from build123d import *

# Parameters (mm, degrees)
SKETCH1_W           = 200
SKETCH1_H           = 100
BOSS_EXTRUDE1_DEPTH = 20
SKETCH2_R           = 7.5
CUT_EXTRUDE1_DEPTH  = 20
BOSS_EXTRUDE2_DEPTH = 10
SKETCH4_R           = 7.5
CUT_EXTRUDE2_DEPTH  = 20


with BuildPart() as part:
    # Sketch1 → Boss-Extrude1 (new body)
    with BuildSketch(Plane(origin=(0, 0, 0), x_dir=(1, 0, 0), z_dir=(0, 1, 0))):
        Rectangle(SKETCH1_W, SKETCH1_H)
    extrude(amount=BOSS_EXTRUDE1_DEPTH)

    # Sketch2 → Cut-Extrude1 (cut)
    with BuildSketch(Plane(origin=(0, 20, 0), x_dir=(1, 0, 0), z_dir=(0, 1, 0))):
        with Locations((-75, 30)):
            Circle(SKETCH2_R)
        with Locations((-25, 30)):
            Circle(SKETCH2_R)
        with Locations((25, 30)):
            Circle(SKETCH2_R)
        with Locations((75, 30)):
            Circle(SKETCH2_R)
        with Locations((-75, -30)):
            Circle(SKETCH2_R)
        with Locations((-25, -30)):
            Circle(SKETCH2_R)
        with Locations((25, -30)):
            Circle(SKETCH2_R)
        with Locations((75, -30)):
            Circle(SKETCH2_R)
    extrude(amount=-CUT_EXTRUDE1_DEPTH, mode=Mode.SUBTRACT)

    # Sketch3 → Boss-Extrude2 (add, symmetric)
    with BuildSketch(Plane.XY):
        with BuildLine():
            Line((-100, 20), (100, 20))
            Line((100, 20), (157.3406431, 60.150350545))
            ThreePointArc((157.3406431, 60.150350545), (161.735357089, 79.923793338), (142.426691144, 86.045718717))
            Line((142.426691144, 86.045718717), (15.876102092, 27.36202298))
            ThreePointArc((15.876102092, 27.36202298), (0, 37.5), (-15.876102092, 27.36202298))
            Line((-15.876102092, 27.36202298), (-142.426691144, 86.045718717))
            ThreePointArc((-142.426691144, 86.045718717), (-161.735357089, 79.923793338), (-157.3406431, 60.150350545))
            Line((-157.3406431, 60.150350545), (-100, 20))
        make_face()
    extrude(amount=BOSS_EXTRUDE2_DEPTH, both=True)

    # Sketch4 → Cut-Extrude2 (cut)
    with BuildSketch(Plane.XY.offset(10)):
        with Locations((148.736996555, 72.437631209)):
            Circle(SKETCH4_R)
        with Locations((-148.736996555, 72.437631209)):
            Circle(SKETCH4_R)
    extrude(amount=-CUT_EXTRUDE2_DEPTH, mode=Mode.SUBTRACT)


solid = part.part
Can you work these out from the model? Positions are in its coordinate system, mm. A direction names the side the tool comes from. Coordinates: 2 decimals unless noted, no trailing zeros. Write each loop counter-clockwise with the first axis right and the second up, starting at its lowest first coordinate (ties: lowest second). Pieces come first, ordered by that corner, then holes. Notation, with made-up numbers: M -34.5,-2 L -0.5,-2 A31 cw -0.5,22 Z; hole C 11,-37.5 d2. An arc over 180 degrees is marked long. Use one line per item in the form item = value.
Q1. If we section it at D-D (x = -75): Write out the boundary of the cut face in (y, z), then the cut area to 3 significant figures.
Model answer:
outline = M 0,-50 L 20,-50 L 20,-37.5 L 0,-37.5 Z; M 0,-22.5 L 20,-22.5 L 20,-10 L 54.78,-10 L 54.78,10 L 20,10 L 20,22.5 L 0,22.5 Z; M 0,37.5 L 20,37.5 L 20,50 L 0,50 Z
area = 2,100 mm^2
Q2. We'd pull the mould along X, two halves only. Please class faces 6 (the cylindrical face through (-30.952, 10.14, 34.564)), 7 (the flat face through (-1, 10, 50)), 8 (the flat face through (128.269, 39.794, 0.14)), 9 (the cylindrical face through (-80.952, 10.14, -25.436)): +X half, -X half, draft (parallel to the pull), parting line (faces both ways), or undercut.
Model answer:
face_6 = undercut
face_7 = draft
face_8 = +X half
face_9 = undercut
Q3. If we section it at A-A (z = 30): Write out the boundary of the cut face in (x, y), then the cut area to 3 significant figures.
Model answer:
outline = M -100,0 L -82.5,0 L -82.5,20 L -100,20 Z; M -67.5,0 L -32.5,0 L -32.5,20 L -67.5,20 Z; M -17.5,0 L 17.5,0 L 17.5,20 L -17.5,20 Z; M 32.5,0 L 67.5,0 L 67.5,20 L 32.5,20 Z; M 82.5,0 L 100,0 L 100,20 L 82.5,20 Z
area = 2,800 mm^2
Q4. If we section it at C-C (x = 41): Write out the boundary of the cut face in (y, z), then the cut area to 3 significant figures.
Model answer:
outline = M 0,-50 L 20,-50 L 20,-10 L 39.01,-10 L 39.01,10 L 20,10 L 20,50 L 0,50 Z
area = 2,380 mm^2
Q5. For P1, Ø5, axis at x = -110.5, y = 30, coming from the +Z side; P2, Ø24, axis at x = 25, z = -30, coming from the +Y side; P3, Ø6, axis at y = 55.5, z = 4, coming from the -X side; P4, Ø13.5, axis at x = -75, z = -30, coming from the -Y side, each with a flat end and sliding along its axis, tell me the tip position at first contact or that it passes through.
Model answer:
P1 = 10
P2 = 20
P3 = -154.98
P4 = through
Q6. For faces 1 (the flat face through (80.037, 57.115, 0.14)), 2 (the flat face through (-1, 0, -1)), 3 (the flat face through (-2, 32, 10)), 4 (the cylindrical face through (69.048, 10.14, -25.436)), 5 (the flat face through (-1, 20, -30)), which set-ups out of +Z, -Z, +X, -X, +Y, -Y let a thin tool reach every point of the face, with its end or its side?
Model answer:
face_1 = +Z, -Z, +Y
face_2 = +Z, -Z, +X, -X, -Y
face_3 = +Z, +X, -X, +Y
face_4 = +Y, -Y
face_5 = -Z, +X, -X, +Y
Q7. If we section it at B-B (x = -25): Write out the boundary of the cut face in (y, z).
Model answer:
outline = M 0,-50 L 20,-50 L 20,-37.5 L 0,-37.5 Z; M 0,-22.5 L 20,-22.5 L 20,-10 L 31.59,-10 L 31.59,10 L 20,10 L 20,22.5 L 0,22.5 Z; M 0,37.5 L 20,37.5 L 20,50 L 0,50 Z
Q8. I need wall thicknesses on line 1 along Z through (x, y) = (-75, 8.5); line 2 along X through (y, z) = (13.25, -30); line 3 along Z through (x, y) = (78.5, 16.5). Which ranges of each line are inside material? Lowest first, please. Write a range as from..to.
Model answer:
line_1 = -50..-37.5, -22.5..22.5, 37.5..50
line_2 = -100..-82.5, -67.5..-32.5, -17.5..17.5, 32.5..67.5, 82.5..100
line_3 = -50..-36.63, -23.37..23.37, 36.63..50
